```python
from build123d import *

# Parameters (mm, degrees)
DODANIE_WYCI_GNI_CIE1_DEPTH = 2
SZKIC2_W                    = 5
SZKIC2_H                    = 16
WYTNIJ_WYCI_GNI_CIE1_DEPTH  = 5
WYTNIJ_WYCI_GNI_CIE2_DEPTH  = 10


with BuildPart() as part:
    # Szkic1 → Dodanie-wyciągnięcie1 (new body)
    with BuildSketch(Plane.XY):
        Polygon((39.660703644, 7.348041155), (39.998203889, -8.651958845), (67.367690874, -8.651958845), (67.367690874, 7.348041155), align=None)
    extrude(amount=-DODANIE_WYCI_GNI_CIE1_DEPTH)

    # Szkic2 → Wytnij-wyciągnięcie1 (cut)
    with BuildSketch(Plane.XY):
        with Locations((64.867690874, -0.651958845)):
            Rectangle(SZKIC2_W, SZKIC2_H)
    extrude(amount=-WYTNIJ_WYCI_GNI_CIE1_DEPTH, mode=Mode.SUBTRACT)

    # Szkic3 → Wytnij-wyciągnięcie2 (cut)
    with BuildSketch(Plane.XY):
        with BuildLine():
            Line((39.660703644, 7.348041155), (39.998203889, -8.651958845))
            Line((39.998203889, -8.651958845), (48.125210145, -8.651958845))
            ThreePointArc((48.125210145, -8.651958845), (51.694710699, -0.869414217), (49.289973229, 7.348041155))
            Line((49.289973229, 7.348041155), (39.660703644, 7.348041155))
        make_face()
    extrude(amount=-WYTNIJ_WYCI_GNI_CIE2_DEPTH, mode=Mode.SUBTRACT)


solid = part.part
```
CAD build for the part. Positions are in the model's coordinates, mm. Coordinates: 2 decimals unless noted, no trailing zeros. Write each loop counter-clockwise with the first axis right and the second up, starting at its lowest first coordinate (ties: lowest second). Pieces come first, ordered by that corner, then holes. Notation, with made-up numbers: (-33.5, 8) -> (-19.5, 8) arc R20 ccw to (-19.5, 28) -> close; hole circle Ø9 at (-27, -31). An arc over 180 degrees is marked (long way). Use CSV: the item, a comma, the result in double quotes. Start each with the question number.
Item 1: Band-saw the part on A-A, the plane z = -0.8. Write the cut outline in (x, y), plus the area to 3 significant figures.
Item 2: Two-plate mould, pull along Y, no slides. Class faces 1 (the flat face through (57, -1, -2)), 2 (the flat face through (55, -8.652, -1)), 3 (the cylindrical face through (51.685, -0.992, -0.986)): +Y half, -Y half, draft (parallel to the pull), parting line (faces both ways), or undercut.
Item 3: Band-saw the part on B-B, the plane y = 3.5. Write the cut outline in (x, z), plus the area to 3 significant figures.
Item 4: Wall check: probe 1 along X at (y, z) = (0, -0.55); probe 2 along X at (y, z) = (-2.5, -0.3). Give the ranges that are in metal, low to high.
Response values:
1,outline,"(48.13, -8.65) -> (62.37, -8.65) -> (62.37, 7.35) -> (49.29, 7.35) arc R12.24 cw to start"
1,area,"186 mm2"
2,face 1,"draft"
2,face 2,"-Y half"
2,face 3,"undercut"
3,outline,"(51.22, -2) -> (62.37, -2) -> (62.37, 0) -> (51.22, 0) -> close"
3,area,"22.3 mm2"
4,probe 1,"x = 51.73 to 62.37"
4,probe 2,"x = 51.46 to 62.37"
